Design review of the part built by this model. Coordinates are the model's own, in mm. Coordinates: 2 decimals unless noted, no trailing zeros. Write each question's results on one line, items separated by ' | '. Start each with the question number.
```python
from build123d import *

# Parameters (mm, degrees)
SKETCH2_R           = 38.1
BOSS_EXTRUDE1_DEPTH = 2.54
BOSS_EXTRUDE2_DEPTH = 12.7
SKETCH4_R           = 1.524
CUT_EXTRUDE1_DEPTH  = 3.81
CUT_EXTRUDE2_DEPTH  = 46.228


with BuildPart() as part:
    # Sketch2 → Boss-Extrude1 (new body)
    with BuildSketch(Plane.XY):
        Circle(SKETCH2_R)
    extrude(amount=BOSS_EXTRUDE1_DEPTH)

    # Sketch3 → Boss-Extrude2 (add)
    with BuildSketch(Plane.XY.offset(2.54)):
        with BuildLine():
            ThreePointArc((-37.360397619, 7.470655243), (-38.1, 0), (-37.360397619, -7.470655243))
            add(Edge.make_bspline(
                [(-25.149976033, -28.619725812), (14.41186903, 8.320696464), (-37.360397619, -7.470655243)],
                knots=[0, 0, 0, 1, 1, 1], degree=2))
            ThreePointArc((-25.149976033, -28.619725812), (-19.05, -32.995567884), (-12.210421586, -36.090381055))
            add(Edge.make_bspline(
                [(12.210421586, -36.090381055), (0, 16.641392928), (-12.210421586, -36.090381055)],
                knots=[0, 0, 0, 1, 1, 1], degree=2))
            ThreePointArc((12.210421586, -36.090381055), (19.05, -32.995567884), (25.149976033, -28.619725812))
            add(Edge.make_bspline(
                [(37.360397619, -7.470655243), (-14.41186903, 8.320696464), (25.149976033, -28.619725812)],
                knots=[0, 0, 0, 1, 1, 1], degree=2))
            ThreePointArc((37.360397619, -7.470655243), (38.1, 0), (37.360397619, 7.470655243))
            add(Edge.make_bspline(
                [(25.149976033, 28.619725812), (-14.41186903, -8.320696464), (37.360397619, 7.470655243)],
                knots=[0, 0, 0, 1, 1, 1], degree=2))
            ThreePointArc((25.149976033, 28.619725812), (19.05, 32.995567884), (12.210421586, 36.090381055))
            add(Edge.make_bspline(
                [(-12.210421586, 36.090381055), (0, -16.641392928), (12.210421586, 36.090381055)],
                knots=[0, 0, 0, 1, 1, 1], degree=2))
            ThreePointArc((-12.210421586, 36.090381055), (-19.05, 32.995567884), (-25.149976033, 28.619725812))
            add(Edge.make_bspline(
                [(-37.360397619, 7.470655243), (14.41186903, -8.320696464), (-25.149976033, 28.619725812)],
                knots=[0, 0, 0, 1, 1, 1], degree=2))
        make_face()
    extrude(amount=BOSS_EXTRUDE2_DEPTH)

    # Sketch4 → Cut-Extrude1 (cut)
    with BuildSketch(Plane(origin=(0, 0, 0), x_dir=(-1, 0, 0), z_dir=(0, 0, -1))):
        Circle(SKETCH4_R)
    extrude(amount=-CUT_EXTRUDE1_DEPTH, mode=Mode.SUBTRACT)

    # Sketch6 → Cut-Extrude2 (cut)
    with BuildSketch(Plane.XY.offset(15.24)):
        with BuildLine():
            ThreePointArc((25.149976033, -28.619725812), (32.995567884, -19.05), (37.360397619, -7.470655243))
            add(Edge.make_bspline(
                [(25.149976033, -28.619725812), (-14.41186903, 8.320696464), (37.360397619, -7.470655243)],
                knots=[0, 0, 0, 1, 1, 1], degree=2))
        make_face()
        with BuildLine():
            ThreePointArc((37.360397619, 7.470655243), (32.995567884, 19.05), (25.149976033, 28.619725812))
            add(Edge.make_bspline(
                [(37.360397619, 7.470655243), (-14.41186903, -8.320696464), (25.149976033, 28.619725812)],
                knots=[0, 0, 0, 1, 1, 1], degree=2))
        make_face()
        with BuildLine():
            ThreePointArc((12.210421586, 36.090381055), (0, 38.1), (-12.210421586, 36.090381055))
            add(Edge.make_bspline(
                [(12.210421586, 36.090381055), (0, -16.641392928), (-12.210421586, 36.090381055)],
                knots=[0, 0, 0, 1, 1, 1], degree=2))
        make_face()
        with BuildLine():
            ThreePointArc((-25.149976033, 28.619725812), (-32.995567884, 19.05), (-37.360397619, 7.470655243))
            add(Edge.make_bspline(
                [(-25.149976033, 28.619725812), (14.41186903, -8.320696464), (-37.360397619, 7.470655243)],
                knots=[0, 0, 0, 1, 1, 1], degree=2))
        make_face()
        with BuildLine():
            ThreePointArc((-37.360397619, -7.470655243), (-32.995567884, -19.05), (-25.149976033, -28.619725812))
            add(Edge.make_bspline(
                [(-37.360397619, -7.470655243), (14.41186903, 8.320696464), (-25.149976033, -28.619725812)],
                knots=[0, 0, 0, 1, 1, 1], degree=2))
        make_face()
        with BuildLine():
            ThreePointArc((-12.210421586, -36.090381055), (0, -38.1), (12.210421586, -36.090381055))
            add(Edge.make_bspline(
                [(-12.210421586, -36.090381055), (0, 16.641392928), (12.210421586, -36.090381055)],
                knots=[0, 0, 0, 1, 1, 1], degree=2))
        make_face()
    extrude(amount=-CUT_EXTRUDE2_DEPTH, mode=Mode.SUBTRACT)


solid = part.part
```
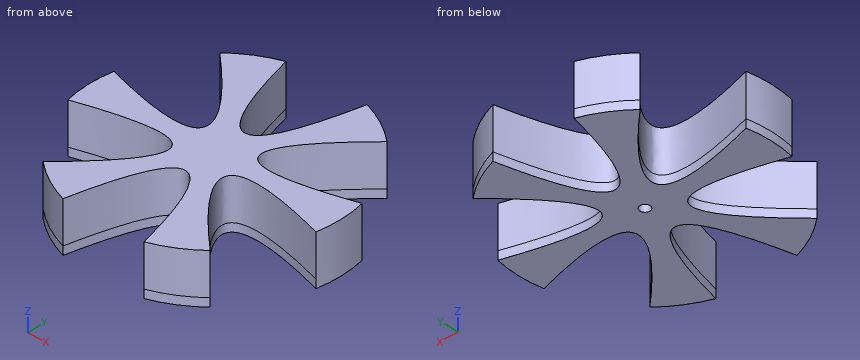
Item 1: Wall thickness on L1, parallel to Y at x = 0, z = 1.75; L2, parallel to Y at x = 12.5, z = 13.5; L3, parallel to X at y = 16.5, z = 7.5: over which ranges is each line inside the solid? List them lowest first.
Item 2: Insertion check: pin 1 Ø5 at (y, z) = (12.5, 2.5) entering from -X; pin 2 Ø10 at (x, y) = (-26, -20.5) entering from -Z; pin 3 Ø1 at (x, z) = (29.5, 11.5) entering from -Y; pin 4 Ø0.9 at (x, y) = (0, 0) entering from -Z. Each pin has a flat end and moves straight along its axis. Give the tip position at first contact, or say it passes through.
Item 3: We need section A-A on x = 20. Count the separate pieces of the cut face and the enclosed holes in it, then the cut area to 3 significant figures.
Answer:
1) L1: y = -9.72 to -1.52, 1.52 to 9.72 | L2: y = -35.99 to -15.35, -2.85 to 2.85, 15.35 to 35.99 | L3: x = -13.43 to -6.19, 6.19 to 13.43
2) pin 1: stops at x = -12.23 | pin 2: passes through | pin 3: stops at y = -5.37 | pin 4: stops at z = 3.81
3) separate pieces: 3 | enclosed holes: 0 | area: 366 mm^2
